Autodesk Inventor part; units mm, degrees
ref_plane "YZ Plane" through (0, 0, 0) normal (1, 0, 0) x (0, 1, 0)
ref_plane "XZ Plane" through (0, 0, 0) normal (0, 1, 0) x (-1, 0, 0)
ref_plane "XY Plane" through (0, 0, 0) normal (0, 0, 1) x (1, 0, 0)
sketch "Sketch1" plane through (0, 0, 0) normal (0, 1, 0) x (-1, 0, 0)
  circle A0 centre (0, 0) radius 25.4
  dimension "d0" = 50.8
extrude "Extrusion1" add sketch "Sketch1" along normal blind 19.05
sketch "Sketch2" plane through (0, 19.05, 0) normal (0, 1, 0) x (1, 0, 0)
  circle A0 centre (0, 0) radius 15.875
  dimension "d3" = 31.75
extrude "Extrusion2" add sketch "Sketch2" along normal blind 6.35
sketch "Sketch3" plane through (0, 25.4, 0) normal (0, 1, 0) x (1, 0, 0)
  circle A0 centre (0, 0) radius 4.7625
  dimension "d6" = 9.525
extrude "Extrusion3" cut sketch "Sketch3" along normal blind 31.75
sketch "Sketch4" plane through (0, 25.4, 0) normal (0, 1, 0) x (1, 0, 0)
  circle A0 centre (0, 0) radius 4.7625
  dimension "d9" = 9.525
extrude "Extrusion4" cut sketch "Sketch4" against normal blind 31.75
properties part number "2 inch Diameter Belt Gear"
Here's how the part is built. I have some questions about the finished solid (model axes, mm). A direction names the side the tool comes from. Give positions to 0.01 mm unless a question says otherwise; leave off trailing zeros. Loops run counter-clockwise (first coordinate to the right, second up) from the corner with the lowest first, then second, coordinate; pieces in that order, holes last. Notation, with made-up numbers: M 54,70 L 88,70 A30 ccw 88,98 Z; hole C 62.25,87.25 d6. An arc over 180 degrees is marked long. Use one line per item in the form item = value. Start each with the question number.
Q1. Will these pins go through, and if not, where does the flat tip stop? pin 1 Ø10 at (x, z) = (7, 12.5) entering from -Y; pin 2 Ø1.5 at (x, y) = (-2.5, 2.5) entering from +Z; pin 3 Ø4 at (y, z) = (10, 13.5) entering from +X; pin 4 Ø3 at (x, y) = (-4, 21.5) entering from -Z.
Q2. I need wall thicknesses on line 1 along Z through (x, y) = (0, 16.25); line 2 along X through (y, z) = (19.75, 0) (1 decimal); line 3 along Y through (x, z) = (22.5, -2.5). Which ranges of each line are inside material? Lowest first, please.
Q3. Thinking about a two-plate mould opening in X: for faces 1 (the cylindrical face through (-3.78, 12.88, 2.9)), 2 (the cylindrical face through (-3.441, 22.181, -15.497)), 3 (the flat face through (3, 25.4, -4)), which applies, +X half, -X half, draft (parallel to the pull), parting line (faces both ways), or undercut?
Q4. If we section it at D-D (z = 6): Write out the boundary of the cut face in (x, y), then the cut area to 3 significant figures.
Q5. If we section it at B-B (z = -3): Write out the boundary of the cut face in (x, y).
Q6. Which directions (+Z, -Z, +X, -X, +Y, -Y) give clear straight access to the entire face, cutting with the end or side of a thin tool? Please do faces 4 (the cylindrical face through (5.506, 9.392, 24.796)), 5 (the flat face through (12, 19.05, -11)).
Q7. If we section it at C-C (y = 17.5): Write out the boundary of the cut face in (x, z) (1 decimal).
Taken from the geometry:
q1.pin_1 = 0
q1.pin_2 = 25.34
q1.pin_3 = 22.65
q1.pin_4 = -15.68
q2.line_1 = -25.4 to -4.76, 4.76 to 25.4
q2.line_2 = -15.9 to -4.8, 4.8 to 15.9
q2.line_3 = 0 to 19.05
q3.face_1 = undercut
q3.face_2 = parting line
q3.face_3 = draft
q4.outline = M -24.68,0 L 24.68,0 L 24.68,19.05 L 14.7,19.05 L 14.7,25.4 L -14.7,25.4 L -14.7,19.05 L -24.68,19.05 Z
q4.area = 1,130 mm^2
q5.outline = M -25.22,0 L -3.7,0 L -3.7,25.4 L -15.59,25.4 L -15.59,19.05 L -25.22,19.05 Z; M 3.7,0 L 25.22,0 L 25.22,19.05 L 15.59,19.05 L 15.59,25.4 L 3.7,25.4 Z
q6.face_4 = +Y, -Y
q6.face_5 = +Y
q7.outline = C 0,0 d50.8; hole C 0,0 d9.5
